```python
from build123d import *

# Parameters (mm, degrees)
SKETCH1_R               = 34.5
BOSS_EXTRUDE1_DEPTH     = 4.5
SKETCH2_W               = 2.65
SKETCH2_H               = 2
CUT_EXTRUDE1_DEPTH      = 49.997448913
CUT_EXTRUDE1_DEPTH_BACK = 49.997448913
SKETCH4_W               = 1.55
SKETCH4_H               = 1.5


with BuildPart() as part:
    # Sketch1 → Boss-Extrude1 (new body)
    with BuildSketch(Plane.XY):
        Circle(SKETCH1_R)
    extrude(amount=BOSS_EXTRUDE1_DEPTH)

    # Sketch2 → Cut-Revolve1 (revolve, cut)
    with BuildSketch(Plane(origin=(0, 0, 0), x_dir=(1, 0, 0), z_dir=(0, 1, 0)), mode=Mode.PRIVATE) as cut_revolve1_sk:
        with Locations((33.175, -1)):
            Rectangle(SKETCH2_W, SKETCH2_H)
    revolve(cut_revolve1_sk.sketch.rotate(Axis((0, 0, 0), (0, 0, 1)), 180), axis=Axis((0, 0, 0), (0, 0, 1)), mode=Mode.SUBTRACT)

    # Sketch4 → Cut-Extrude1 (cut, two sides: drawn at the far end of the back side and taken through both)
    with BuildSketch(Plane(origin=(0, 0, 0), x_dir=(1, 0, 0), z_dir=(0, 1, 0)).offset(-CUT_EXTRUDE1_DEPTH_BACK)):
        with Locations((0, -0.75)):
            Rectangle(SKETCH4_W, SKETCH4_H)
    extrude(amount=CUT_EXTRUDE1_DEPTH + CUT_EXTRUDE1_DEPTH_BACK, mode=Mode.SUBTRACT)


solid = part.part
```
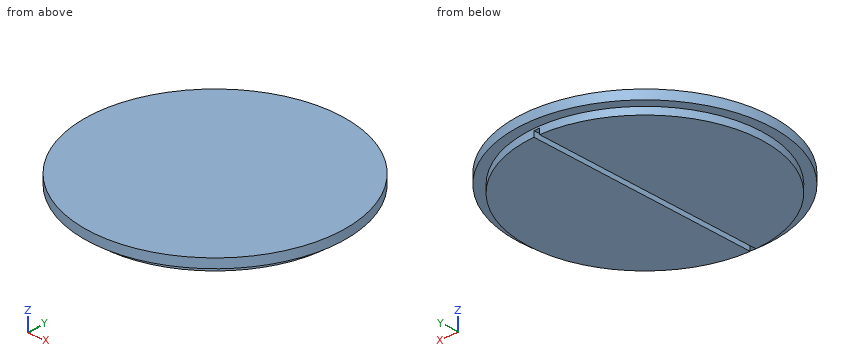
Model file for the job. Use its own axes, mm. Round coordinates to 2 decimals unless told otherwise and drop trailing zeros. Write each loop counter-clockwise with the first axis right and the second up, starting at its lowest first coordinate (ties: lowest second). Pieces come first, ordered by that corner, then holes. Notation, with made-up numbers: (45, 38) - (82, 38) arc R6 ccw to (82, 45) - close; hole circle Ø2 at (84, -36.75). An arc over 180 degrees is marked (long way). One line per item, written item: value.
(1) Drop flat-ended pins along their axis: P1, Ø1, axis at x = -9.5, y = -23, coming from the -Z side; P2, Ø1.6, axis at y = 8.5, z = 1, coming from the -X side; P3, Ø2, axis at x = -20, z = 1.5, coming from the -Y side; P4, Ø1.2, axis at x = 0, y = -7.5, coming from the -Z side. Give the stop position or say it passes through.
Values follow:
P1: stops at z = 0
P2: stops at x = -30.91
P3: stops at y = -28.71
P4: stops at z = 1.5
(2) Cut at A-A, the plane z = 0.7. Give the cut face in (x, y) (3 decimals).
Values follow:
outline: (-0.775, -31.841) - (-0.775, 31.841) arc R31.85 ccw to start; (0.775, -31.841) arc R31.85 ccw to (0.775, 31.841) - close
(3) Cut at C-C, the plane x = 19. Give the cut face in (y, z), plus the area to 3 significant figures.
Values follow:
outline: (-28.8, 2) - (-25.56, 2) - (-25.56, 0) - (25.56, 0) - (25.56, 2) - (28.8, 2) - (28.8, 4.5) - (-28.8, 4.5) - close
area: 246 mm²
(4) Wall check: probe 1 along Z at (x, y) = (22, -24); probe 2 along X at (y, z) = (12, 0.6) (3 decimals); probe 3 along X at (y, z) = (4.5, 0.3) (1 decimal). Give the ranges that are in metal, low to high.
Values follow:
probe 1: z = 2 to 4.5
probe 2: x = -29.503 to -0.775, 0.775 to 29.503
probe 3: x = -31.5 to -0.8, 0.8 to 31.5
(5) Cut at D-D, the plane x = 6. Give the cut face in (y, z).
Values follow:
outline: (-33.97, 2) - (-31.28, 2) - (-31.28, 0) - (31.28, 0) - (31.28, 2) - (33.97, 2) - (33.97, 4.5) - (-33.97, 4.5) - close
(6) Cut at B-B, the plane y = 0. Give the cut face in (x, z) (3 decimals).
Values follow:
outline: (-34.5, 2) - (-31.85, 2) - (-31.85, 0) - (-0.775, 0) - (-0.775, 1.5) - (0.775, 1.5) - (0.775, 0) - (31.85, 0) - (31.85, 2) - (34.5, 2) - (34.5, 4.5) - (-34.5, 4.5) - close
